from build123d import *

# Parameters (mm, degrees)
EXTRUDE_THIN1_DEPTH = 10
EXTRUDE1_DEPTH      = 0.35


with BuildPart() as part:
    # Sketch1 → Extrude-Thin1 (new body)
    with BuildSketch(Plane(origin=(0, 0, 0), x_dir=(1, 0, 0), z_dir=(0, 1, 0))):
        with BuildLine():
            ThreePointArc((-0.75, -1.854049622), (-1.954040628, -0.426292414), (-1.454057939, 1.373213571))
            ThreePointArc((-1.454057939, 1.373213571), (-1.255350091, 1.512238811), (-1.017840557, 1.5612495))
            Line((-1.017840557, 1.5612495), (1.017840557, 1.5612495))
            ThreePointArc((1.017840557, 1.5612495), (1.255350091, 1.512238811), (1.454057939, 1.373213571))
            ThreePointArc((1.454057939, 1.373213571), (1.954040628, -0.426292414), (0.75, -1.854049622))
            Line((0.75, -1.854049622), (0.61875, -1.529590938))
            ThreePointArc((0.61875, -1.529590938), (1.612083519, -0.351691242), (1.199597799, 1.132901196))
            ThreePointArc((1.199597799, 1.132901196), (1.116802863, 1.190828379), (1.017840557, 1.2112495))
            Line((1.017840557, 1.2112495), (-1.017840557, 1.2112495))
            ThreePointArc((-1.017840557, 1.2112495), (-1.116802863, 1.190828379), (-1.199597799, 1.132901196))
            ThreePointArc((-1.199597799, 1.132901196), (-1.612083519, -0.351691242), (-0.61875, -1.529590938))
            Line((-0.61875, -1.529590938), (-0.75, -1.854049622))
        make_face()
    extrude(amount=EXTRUDE_THIN1_DEPTH)

    # Sketch2 → Extrude1 (add)
    with BuildSketch(Plane.XY.offset(-1.2112495)):
        with BuildLine():
            Line((-1, 0), (-1, -1))
            Line((-1, -1), (-2, -2))
            Line((-2, -2), (-2, -9))
            ThreePointArc((-2, -9), (0, -11), (2, -9))
            Line((2, -9), (2, -2))
            Line((2, -2), (1, -1))
            Line((1, -1), (1, 0))
            Line((1, 0), (-1, 0))
        make_face()
        with BuildLine():
            Line((0.9, -9), (0.9, -6.5))
            ThreePointArc((0.9, -6.5), (0, -5.6), (-0.9, -6.5))
            Line((-0.9, -6.5), (-0.9, -9))
            ThreePointArc((-0.9, -9), (0, -9.9), (0.9, -9))
        make_face(mode=Mode.SUBTRACT)
    extrude(amount=-EXTRUDE1_DEPTH)


solid = part.part
Check sheet for the modelled part. Datum: model origin and axes. Units: mm. A direction names the side the tool comes from. Round coordinates to 2 decimals unless told otherwise and drop trailing zeros. Order: outer loops, then holes, each group sorted by start corner. A loop starts at its lowest first (then second) coordinate and runs counter-clockwise, first axis right, second up.
(1) Access from +Z, -Z, +X, -X, +Y, -Y to the whole of each face (thin tool, end or side, straight path). Record for faces 4 (the flat face through (1.5, -1.5, -1.4)), 5 (the cylindrical face through (1.6, 4.9, 0.4)), 6 (the flat face through (-1.5, -1.5, -1.4)).
(2) Cross-section at D-D, the plane y = -2.5. Enter the section's corners in (x, z).
(3) Cross-section at B-B, the plane y = -8.5. Enter the section's corners in (x, z), and give its area (3 significant figures).
(4) Go/stop test with flat-tipped pins: P1, Ø1, axis at x = 1, y = 7.5, coming from the +Z side; P2, Ø0.7, axis at x = -1.5, z = 0, coming from the -Y side; P3, Ø1, axis at y = -5.5, z = 0, coming from the -X side; P4, Ø1, axis at x = -0.5, y = -6, coming from the +Z side. Record where each tip stops, or that it passes through.
(5) Draft check along Y on faces 1 (the cylindrical face through (0, -11, -1.4)), 2 (the cylindrical face through (-2, 5, 0)), 3 (the cylindrical face through (0, -5.6, -1.4)). Enter one of: pulls with the +Y half, pulls with the -Y half, needs draft (parallel to the pull), parting line crosses it, or undercut.
(6) Scan lines: probe 1 along X at (y, z) = (4.5, 0); probe 2 along Y at (x, z) = (1.5, 1); probe 3 along Z at (x, y) = (-1.05, -3). Record each from-to range of solid material in increasing order.
(7) Cross-section at A-A, the plane x = 0. Enter the section's corners in (y, z).
(8) Cross-section at C-C, the plane y = 4.25. Enter the section's corners in (x, z), and give its area (3 significant figures).
Check sheet entries:
1. face 4: +Z, -Z, +X
1. face 5: +Y, -Y
1. face 6: +Z, -Z, -X
2. outline: (-2, -1.56) - (2, -1.56) - (2, -1.21) - (-2, -1.21) - close
3. outline: (-2, -1.56) - (-0.9, -1.56) - (-0.9, -1.21) - (-2, -1.21) - close; (0.9, -1.56) - (2, -1.56) - (2, -1.21) - (0.9, -1.21) - close
3. area: 0.770 mm2
4. P1: stops at z = 1.85
4. P2: stops at y = 0
4. P3: passes through
4. P4: stops at z = -1.21
5. face 1: pulls with the -Y half
5. face 2: needs draft
5. face 3: undercut
6. probe 1: x = -2 to -1.65, 1.65 to 2
6. probe 2: y = 0 to 10
6. probe 3: z = -1.56 to -1.21
7. outline: (-11, -1.56) - (-9.9, -1.56) - (-9.9, -1.21) - (-11, -1.21) - close; (-5.6, -1.56) - (10, -1.56) - (10, -1.21) - (-5.6, -1.21) - close
8. outline: (-1.45, -1.37) arc R0.6 ccw to (-1.02, -1.56) - (1.02, -1.56) arc R0.6 ccw to (1.45, -1.37) arc R2 ccw to (0.75, 1.85) - (0.62, 1.53) arc R1.65 cw to (1.2, -1.13) arc R0.25 cw to (1.02, -1.21) - (-1.02, -1.21) arc R0.25 cw to (-1.2, -1.13) arc R1.65 cw to (-0.62, 1.53) - (-0.75, 1.85) arc R2 ccw to start
8. area: 3.44 mm2
